from build123d import *

# Parameters (mm, degrees)
SKETCH1_R               = 4.5
SKETCH1_R_2             = 1.25
BOSS_EXTRUDE1_DEPTH     = 8
SKETCH2_R               = 1.75
SKETCH2_R_2             = 1.25
CUT_EXTRUDE1_DEPTH      = 4
SKETCH4_W               = 12
SKETCH4_H               = 12
SKETCH4_W_2             = 6.5
SKETCH4_H_2             = 6.5
BOSS_EXTRUDE2_DEPTH     = 12
SKETCH5_W               = 12
SKETCH5_H               = 12
BOSS_EXTRUDE3_DEPTH     = 8
CUT_EXTRUDE2_DEPTH      = 23
CUT_EXTRUDE2_DEPTH_BACK = 23
SKETCH6_R               = 1.1
FILLET1_R               = 2
SKETCH1_2_R             = 4.5
SKETCH1_2_R_2           = 1.25
CUT_EXTRUDE5_DEPTH      = 8
CUT_EXTRUDE6_DEPTH      = 13


with BuildPart() as part:
    # Sketch1 → Boss-Extrude1 (new body)
    with BuildSketch(Plane.XY):
        Circle(SKETCH1_R)
        Circle(SKETCH1_R_2, mode=Mode.SUBTRACT)
    extrude(amount=BOSS_EXTRUDE1_DEPTH)

    # Sketch2 → Cut-Extrude1 (cut)
    with BuildSketch(Plane(origin=(0, 0, 0), x_dir=(-1, 0, 0), z_dir=(0, 0, -1))):
        Circle(SKETCH2_R)
        Circle(SKETCH2_R_2, mode=Mode.SUBTRACT)
    extrude(amount=-CUT_EXTRUDE1_DEPTH, mode=Mode.SUBTRACT)

    # Sketch4 → Boss-Extrude2 (add)
    with BuildSketch(Plane(origin=(0, 0, 0), x_dir=(-1, 0, 0), z_dir=(0, 0, -1))):
        Rectangle(SKETCH4_W, SKETCH4_H)
        Rectangle(SKETCH4_W_2, SKETCH4_H_2, mode=Mode.SUBTRACT)
    extrude(amount=BOSS_EXTRUDE2_DEPTH)

    # Sketch5 → Boss-Extrude3 (add)
    with BuildSketch(Plane(origin=(6, 0, 0), x_dir=(0, 0, -1), z_dir=(1, 0, 0))):
        with Locations((6, 0)):
            Rectangle(SKETCH5_W, SKETCH5_H)
    extrude(amount=BOSS_EXTRUDE3_DEPTH)

    # Sketch6 → Cut-Extrude2 (cut, two sides: drawn at the far end of the back side and taken through both)
    with BuildSketch(Plane(origin=(0, 6, 0), x_dir=(1, 0, 0), z_dir=(0, 1, 0)).offset(-CUT_EXTRUDE2_DEPTH_BACK)):
        with Locations(Location((9, 6, 0), (0, 0, 270))):
            Circle(SKETCH6_R)
    extrude(amount=CUT_EXTRUDE2_DEPTH + CUT_EXTRUDE2_DEPTH_BACK, mode=Mode.SUBTRACT)

    # Fillet1
    fillet1_edges = [part.edges().sort_by_distance(p)[0] for p in [
        (-6, -6, -6),
        (-6, 6, -6),
        (14, 6, -6),
        (14, -6, -6),
    ]]
    fillet(fillet1_edges, radius=FILLET1_R)

    # Sketch1<2> → Cut-Extrude5 (cut)
    with BuildSketch(Plane.XY):
        Circle(SKETCH1_2_R)
        Circle(SKETCH1_2_R_2, mode=Mode.SUBTRACT)
    extrude(amount=CUT_EXTRUDE5_DEPTH, mode=Mode.SUBTRACT)

    # Sketch7 → Cut-Extrude6 (cut)
    with BuildSketch(Plane(origin=(0, 6, 0), x_dir=(1, 0, 0), z_dir=(0, 1, 0))):
        with BuildLine():
            ThreePointArc((-1.25, 6), (0, 4.75), (1.25, 6))
            Line((1.25, 6), (-1.25, 6))
        make_face()
        with BuildLine():
            Line((-1.25, 6), (1.25, 6))
            ThreePointArc((1.25, 6), (0, 7.25), (-1.25, 6))
        make_face()
    extrude(amount=-CUT_EXTRUDE6_DEPTH, mode=Mode.SUBTRACT)


solid = part.part
Check sheet for the modelled part. Datum: model origin and axes. Units: mm. A direction names the side the tool comes from. Round coordinates to 2 decimals unless told otherwise and drop trailing zeros. Loops run counter-clockwise (first coordinate to the right, second up) from the corner with the lowest first, then second, coordinate; pieces in that order, holes last. Notation, with made-up numbers: (74.5, -12.75) - (113.5, -12.75) arc R16 ccw to (113.5, -1.75) - close; hole circle Ø9 at (6.25, 23.5). An arc over 180 degrees is marked (long way). Answer as CSV lines item,"result". Start each with the question number.
Item 1: Section check C-C (z = -9.5). Record the boundary of the cut face in (x, y), and give its area (3 significant figures).
Item 2: Section check A-A (y = -1). Record the boundary of the cut face in (x, z), and give its area (3 significant figures).
Item 3: Section check D-D (x = 0). Record the boundary of the cut face in (y, z), and give its area (4 significant figures).
Item 4: Section check B-B (x = 2). Record the boundary of the cut face in (y, z), and give its area (3 significant figures).
Item 5: Release check for a two-part mould opening along Z. For faces 3 (the flat face through (3.25, 0, -6)), 4 (the flat face through (4, 0, 0)), 5 (the cylindrical face through (8.579, -0.084, -4.984)) record: +Z half, -Z half, draft (parallel to the pull), parting line (faces both ways), or undercut.
Item 6: Depth check by flat-ended pin: P1, Ø2, axis at x = 9, z = -6, coming from the +Y side. Enter the tip coordinate at first touch or a pass-through.
Item 7: Set-up check for faces 1 (the cylindrical face through (-5.4, 5.43, -6.08)), 2 (the flat face through (0, 3.25, -4.6)): record each of +Z, -Z, +X, -X, +Y, -Y from which the full face is reachable in a straight line by a thin tool's end or side.
Item 8: Scan lines: line 1 (X direction, y = 0.75, z = -6); line 2 (X direction, y = -0.5, z = -1.5); line 3 (Z direction, x = 0, y = -4.65). Record each from-to range of solid material in increasing order. Write a range as [from, to].
Report:
1,outline,"(-6, -4) arc R2 ccw to (-4, -6) - (12, -6) arc R2 ccw to (14, -4) - (14, 4) arc R2 ccw to (12, 6) - (-4, 6) arc R2 ccw to (-6, 4) - close; hole (-3.25, -3.25) - (3.25, -3.25) - (3.25, 3.25) - (-3.25, 3.25) - close"
1,area,"194 mm2"
2,outline,"(-6, -12) - (-3.25, -12) - (-3.25, 0) - (-6, 0) - close; (3.25, -12) - (14, -12) - (14, 0) - (3.25, 0) - close; hole circle Ø2.2 at (9, -6)"
2,area,"158 mm2"
3,outline,"(-6, -12) - (-3.25, -12) - (-3.25, -7.25) - (-6, -7.25) - close; (-6, -4.75) - (-3.25, -4.75) - (-3.25, 0) - (-6, 0) - close; (3.25, -12) - (6, -12) - (6, -7.25) - (3.25, -7.25) - close; (3.25, -4.75) - (6, -4.75) - (6, 0) - (3.25, 0) - close"
3,area,"52.25 mm2"
4,outline,"(-6, -12) - (-3.25, -12) - (-3.25, 0) - (-6, 0) - close; (3.25, -12) - (6, -12) - (6, 0) - (3.25, 0) - close"
4,area,"66.0 mm2"
5,face 3,"draft"
5,face 4,"+Z half"
5,face 5,"undercut"
6,P1,"passes through"
7,face 1,"+Z, -Z, -X, +Y"
7,face 2,"+Z, -Z"
8,line 1,"x = [-6, -3.25], [3.25, 7.9], [10.1, 14]"
8,line 2,"x = [-6, -3.25], [3.25, 14]"
8,line 3,"z = [-12, -7.25], [-4.75, 0]"
